Answer from the drawing. Dimensions are ordinates in mm from the lowest x, y and z of the part. A direction names the side the tool comes from. Coordinates: 2 decimals unless noted, no trailing zeros. Loops run counter-clockwise (first coordinate to the right, second up) from the corner with the lowest first, then second, coordinate; pieces in that order, holes last. Notation, with made-up numbers: (-37, -5) -> (-1, -5) arc R24 ccw to (-1, 29) -> close; hole circle Ø2 at (41, 4.25). An arc over 180 degrees is marked (long way). Use a Markdown table: item, result.
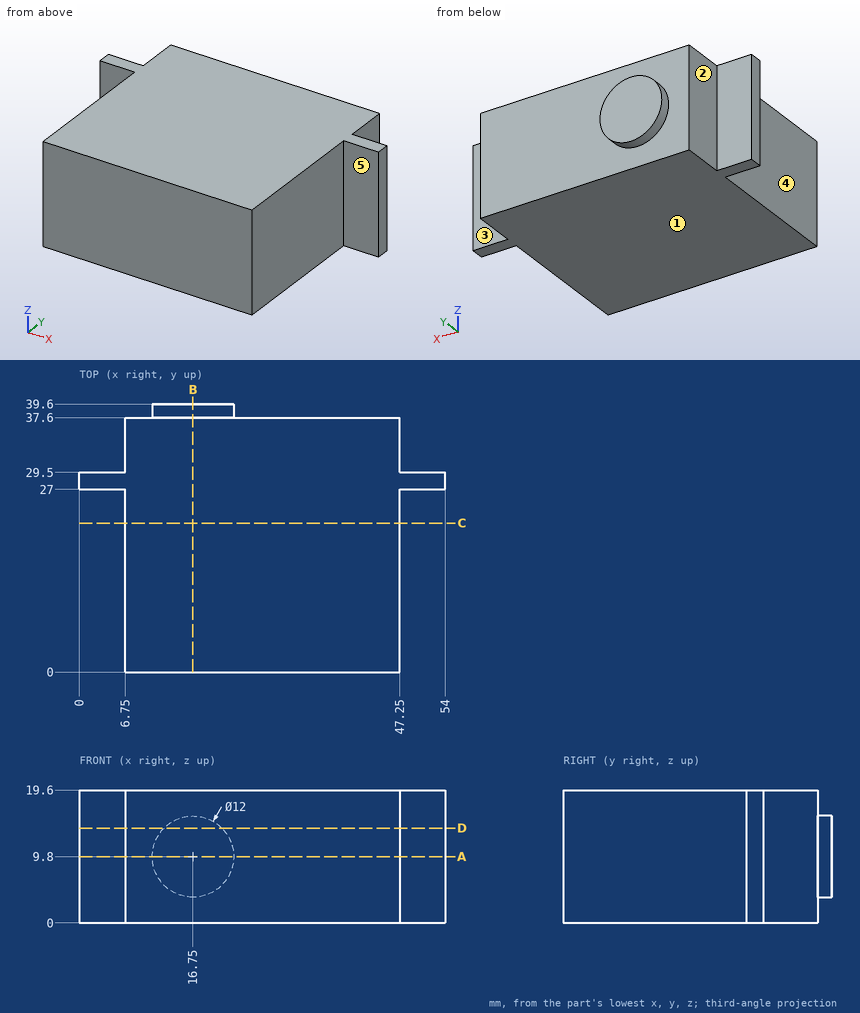
Q1. Section A-A on z = 9.8 is taken. Determine the outline of the cut face in (x, y), and give its area (3 significant figures).
Solved:
| item | result |
|---|---|
| outline | (0, 27) -> (6.75, 27) -> (6.75, 0) -> (47.25, 0) -> (47.25, 27) -> (54, 27) -> (54, 29.5) -> (47.25, 29.5) -> (47.25, 37.6) -> (22.75, 37.6) -> (22.75, 39.6) -> (10.75, 39.6) -> (10.75, 37.6) -> (6.75, 37.6) -> (6.75, 29.5) -> (0, 29.5) -> close |
| area | 1,580 mm² |
Q2. Consider line 1 (Y direction, x = 28, z = 8.5); line 2 (X direction, y = 20.5, z = 7.5); line 3 (Y direction, x = 47.5, z = 11). Determine where each line is inside the solid, lowest interval first. Write a range as [from, to].
Solved:
| item | result |
|---|---|
| line 1 | [0, 37.6] |
| line 2 | [6.75, 47.25] |
| line 3 | [27, 29.5] |
Q3. Section D-D on z = 14 is taken. Determine the outline of the cut face in (x, y), and give its area (3 significant figures).
Solved:
| item | result |
|---|---|
| outline | (0, 27) -> (6.75, 27) -> (6.75, 0) -> (47.25, 0) -> (47.25, 27) -> (54, 27) -> (54, 29.5) -> (47.25, 29.5) -> (47.25, 37.6) -> (21.03, 37.6) -> (21.03, 39.6) -> (12.47, 39.6) -> (12.47, 37.6) -> (6.75, 37.6) -> (6.75, 29.5) -> (0, 29.5) -> close |
| area | 1,570 mm² |
Q4. Section B-B on x = 16.75 is taken. Determine the outline of the cut face in (y, z).
Solved:
| item | result |
|---|---|
| outline | (0, 0) -> (37.6, 0) -> (37.6, 3.8) -> (39.6, 3.8) -> (39.6, 15.8) -> (37.6, 15.8) -> (37.6, 19.6) -> (0, 19.6) -> close |
Q5. Given pin 1 Ø2 at (x, z) = (3, 13) entering from -Y; pin 2 Ø6 at (y, z) = (14, 13.5) entering from -X; pin 3 Ø10 at (y, z) = (13.5, 2.5) entering from +X, each flat-ended and moving along its own axis, determine where each tip first touches the part or whether it passes through.
Solved:
| item | result |
|---|---|
| pin 1 | y = 27 |
| pin 2 | x = 6.75 |
| pin 3 | x = 47.25 |
Q6. Section C-C on y = 22 is taken. Determine the outline of the cut face in (x, z), and give its area (3 significant figures).
Solved:
| item | result |
|---|---|
| outline | (6.75, 0) -> (47.25, 0) -> (47.25, 19.6) -> (6.75, 19.6) -> close |
| area | 794 mm² |
Q7. For the marked faces 1, 2, 3, 4 and 5, determine the directions among +Z, -Z, +X, -X, +Y, -Y from which every point of the face is accessible in a straight line to the end or side of a thin tool.
Solved:
| item | result |
|---|---|
| face 1 | -Z, +X, -X, +Y, -Y |
| face 2 | +Z, -Z, -X, +Y |
| face 3 | +Z, -Z, +X, +Y |
| face 4 | +Z, -Z, -X, -Y |
| face 5 | +Z, -Z, +X, -Y |
